Could you check a few things on this model? Use its own coordinates, in mm. A direction names the side the tool comes from. Give positions to 0.01 mm unless a question says otherwise; leave off trailing zeros. Write each loop counter-clockwise with the first axis right and the second up, starting at its lowest first coordinate (ties: lowest second). Pieces come first, ordered by that corner, then holes. Notation, with made-up numbers: M 28,50 L 78,50 A17 cw 78,58 Z; hole C 80.25,12.25 d1. An arc over 180 degrees is marked long. Answer as a JSON object with one key per item and string values. Group by question number.
```python
from build123d import *

# Parameters (mm, degrees)
SKETCH1_R                  = 95.25
BOSS_EXTRUDE1_DEPTH        = 4.7625
M2X0_4_TAPPED_HOLE1_D      = 1.6
M2X0_4_TAPPED_HOLE1_DEPTH  = 5.334
F_12_24_TAPPED_HOLE1_D     = 4.4958
F_12_24_TAPPED_HOLE1_DEPTH = 14.224
F_10_32_TAPPED_HOLE1_D     = 4.0386
F_10_32_TAPPED_HOLE1_DEPTH = 11.938
SKETCH11_W                 = 99.656274728
SKETCH11_H                 = 17.78
SKETCH11_H_2               = 22.86
SKETCH11_W_2               = 10.59018736
SKETCH11_H_3               = 33.02
SKETCH11_W_3               = 6.264058664
CUT_EXTRUDE2_DEPTH         = 5.7625
SKETCH12_W                 = 80.606274728
SKETCH12_H                 = 139.7
CUT_EXTRUDE3_DEPTH         = 5.7625
FILLET1_R                  = 2.54


with BuildPart() as part:
    # Sketch1 → Boss-Extrude1 (new body)
    with BuildSketch(Plane.XY):
        Circle(SKETCH1_R)
    extrude(amount=BOSS_EXTRUDE1_DEPTH)

    # M2x0.4 Tapped Hole1
    with Locations(Plane.XY.offset(4.7625)):
        with Locations((-84.548324724, 33.02), (-66.768324724, 33.02), (-73.958137364, 50.8), (-56.178137364, 50.8), (-90.812383388, 10.16), (-73.032383388, 10.16), (-56.178137364, -50.8), (-73.958137364, -50.8), (-66.768324724, -33.02), (-84.548324724, -33.02), (-73.032383388, -10.16), (-90.812383388, -10.16), (56.178137364, -50.8), (73.958137364, -50.8), (66.768324724, -33.02), (84.548324724, -33.02), (90.812383388, -10.16), (73.032383388, -10.16), (90.812383388, 10.16), (73.032383388, 10.16), (84.548324724, 33.02), (66.768324724, 33.02), (56.178137364, 50.8), (73.958137364, 50.8)):
            Hole(M2X0_4_TAPPED_HOLE1_D / 2, depth=M2X0_4_TAPPED_HOLE1_DEPTH)

    # #12-24 Tapped Hole1
    with Locations(Plane.XY.offset(4.7625)):
        with Locations((-79.375, 0), (0, 79.375), (79.375, 0), (0, -79.375)):
            Hole(F_12_24_TAPPED_HOLE1_D / 2, depth=F_12_24_TAPPED_HOLE1_DEPTH)

    # #10-32 Tapped Hole1
    with Locations(Plane.XY.offset(4.7625)):
        with Locations((-59.89185243, 63.5), (59.89185243, 63.5)):
            f_10_32_tapped_hole1 = Hole(F_10_32_TAPPED_HOLE1_D / 2, depth=F_10_32_TAPPED_HOLE1_DEPTH)

    # Mirror1: #10-32 Tapped Hole1 across plane
    add(f_10_32_tapped_hole1.mirror(Plane.ZX), mode=Mode.SUBTRACT)

    # Sketch11 → Cut-Extrude2 (cut, through all)
    with BuildSketch(Plane.XY.offset(4.7625)):
        with Locations((0, 48.26)):
            Rectangle(SKETCH11_W, SKETCH11_H)
        with Locations((0, 27.94)):
            Rectangle(SKETCH11_W, SKETCH11_H_2)
        with Locations((-55.123231044, 27.94)):
            Rectangle(SKETCH11_W_2, SKETCH11_H_2)
        with Locations((55.123231044, 27.94)):
            Rectangle(SKETCH11_W_2, SKETCH11_H_2)
        with Locations((55.123231044, 0)):
            Rectangle(SKETCH11_W_2, SKETCH11_H_3)
        with Locations((63.550354056, 0)):
            Rectangle(SKETCH11_W_3, SKETCH11_H_3)
        Rectangle(SKETCH11_W, SKETCH11_H_3)
        with Locations((-55.123231044, 0)):
            Rectangle(SKETCH11_W_2, SKETCH11_H_3)
        with Locations((-63.550354056, 0)):
            Rectangle(SKETCH11_W_3, SKETCH11_H_3)
        with Locations((-55.123231044, -27.94)):
            Rectangle(SKETCH11_W_2, SKETCH11_H_2)
        with Locations((0, -27.94)):
            Rectangle(SKETCH11_W, SKETCH11_H_2)
        with Locations((55.123231044, -27.94)):
            Rectangle(SKETCH11_W_2, SKETCH11_H_2)
        with Locations((0, -48.26)):
            Rectangle(SKETCH11_W, SKETCH11_H)
    extrude(amount=-CUT_EXTRUDE2_DEPTH, mode=Mode.SUBTRACT)

    # Sketch12 → Cut-Extrude3 (cut, through all)
    with BuildSketch(Plane.XY.offset(4.7625)):
        Rectangle(SKETCH12_W, SKETCH12_H)
    extrude(amount=-CUT_EXTRUDE3_DEPTH, mode=Mode.SUBTRACT)

    # Fillet1
    fillet1_edges = [part.edges().sort_by_distance(p)[0] for p in [
        (-49.828137364, 39.37, 2.38125),
        (-49.828137364, 57.15, 2.38125),
        (49.828137364, 57.15, 2.38125),
        (49.828137364, 39.37, 2.38125),
        (60.418324724, 39.37, 2.38125),
        (60.418324724, 16.51, 2.38125),
        (66.682383388, 16.51, 2.38125),
        (66.682383388, -16.51, 2.38125),
        (60.418324724, -16.51, 2.38125),
        (60.418324724, -39.37, 2.38125),
        (49.828137364, -39.37, 2.38125),
        (49.828137364, -57.15, 2.38125),
        (-49.828137364, -57.15, 2.38125),
        (-49.828137364, -39.37, 2.38125),
        (-60.418324724, -39.37, 2.38125),
        (-60.418324724, -16.51, 2.38125),
        (-66.682383388, -16.51, 2.38125),
        (-66.682383388, 16.51, 2.38125),
        (-60.418324724, 16.51, 2.38125),
        (-60.418324724, 39.37, 2.38125),
        (40.303137364, -57.15, 2.38125),
        (-40.303137364, -57.15, 2.38125),
        (-40.303137364, 57.15, 2.38125),
        (40.303137364, 57.15, 2.38125),
        (40.303137364, 69.85, 2.38125),
        (-40.303137364, -69.85, 2.38125),
        (-40.303137364, 69.85, 2.38125),
        (40.303137364, -69.85, 2.38125),
    ]]
    fillet(fillet1_edges, radius=FILLET1_R)


solid = part.part
```
1) If we section it at A-A, the plane y = 22.5: List the corners of the cut face in (x, z) for me, plus the area to 3 significant figures.
2) I'm going to push flat-ended pins straight in: pin 1 (2 mm diameter, centred on y = 30, z = 4, fed in from +X); pin 2 (2 mm diameter, centred on x = 46, z = 1.5, fed in from +Y); pin 3 (2.5 mm diameter, centred on y = 31, z = 2, fed in from +X); pin 4 (1.8 mm diameter, centred on x = -66.77, y = 33.02, fed in from +Z). Where does each tip first touch, or does it pass through?
3) We'd pull the mould along Y, two halves only. Please class faces 3 (the flat face through (62, -20, 0)), 4 (the flat face through (-60.418, -28, 2)): released by +Y, released by -Y, zero draft, split by the parting line, or undercut.
4) If we section it at C-C, the plane z = 2.25: Give the number of separate pieces and of enclosed holes in the cut face, plus the area to 3 significant figures.
5) For faces 1 (the flat face through (62, -20, 4.762)), 2 (the flat face through (60.418, -28, 2)), which set-ups out of +Z, -Z, +X, -X, +Y, -Y let a thin tool reach every point of the face, with its end or its side?
6) Please list where these lines run through material, in increasing order: line 1 along Y through (x, z) = (0, 2.1); line 2 along Y through (x, z) = (-56, 4.45); line 3 along X through (y, z) = (-10.5, 3.1). Write a range as from..to.
7) If we section it at B-B, the plane x = -31.5: List the corners of the cut face in (y, z) for me, plus the area to 3 significant figures.
Taken from the geometry:
{
 "1": {"outline": "M -92.55,0 L -60.42,0 L -60.42,4.76 L -92.55,4.76 Z; M 60.42,0 L 92.55,0 L 92.55,4.76 L 60.42,4.76 Z", "area": "306 mm²"},
 "2": {"pin 1": "x = 90.73", "pin 2": "y = 83.95", "pin 3": "x = 90.48", "pin 4": "z = 4.76"},
 "3": {"face 3": "zero draft", "face 4": "undercut"},
 "4": {"separate pieces": "1", "enclosed holes": "33", "area": "12,800 mm²"},
 "5": {"face 1": "+Z, +X, -X, +Y, -Y", "face 2": "+Z, -Z"},
 "6": {"line 1": "-95.25..-81.62, -77.13..-69.85, 69.85..77.13, 81.62..95.25", "line 2": "-77.05..-51.58, -50.02..-39.37, 39.37..50.02, 51.58..77.05", "line 3": "-94.67..-91.54, -90.09..-73.76, -72.31..-66.68, 66.68..72.31, 73.76..90.09, 91.54..94.67"},
 "7": {"outline": "M -89.89,0 L -69.85,0 L -69.85,4.76 L -89.89,4.76 Z; M 69.85,0 L 89.89,0 L 89.89,4.76 L 69.85,4.76 Z", "area": "191 mm²"}
}
